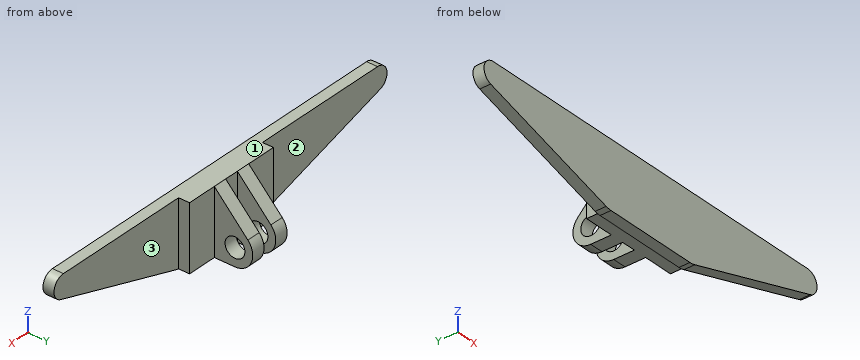
```python
from build123d import *

# Parameters (mm, degrees)
BOSS_EXTRUDE1_DEPTH = 6.9215
FILLET1_R           = 12.7
SKETCH2_W           = 63.5635
SKETCH2_H           = 41.073046068
BOSS_EXTRUDE2_DEPTH = 6.9215
SKETCH3_R           = 6.223
BOSS_EXTRUDE4_DEPTH = 44.7929
SKETCH3_2_R         = 6.223
CUT_EXTRUDE1_DEPTH  = 18.7706
SKETCH4_W           = 8.89
SKETCH4_H           = 24.13
CUT_EXTRUDE2_DEPTH  = 42.2115


with BuildPart() as part:
    # Sketch1 → Boss-Extrude1 (new body)
    with BuildSketch(Plane(origin=(0, 0, 0), x_dir=(1, 0, 0), z_dir=(0, 1, 0))):
        with BuildLine():
            Line((5.071738793, 14.002525941), (94.4245, 41.2115))
            Line((94.4245, 41.2115), (157.988, 41.2115))
            Line((157.988, 41.2115), (247.340761207, 14.002525941))
            ThreePointArc((247.340761207, 14.002525941), (252.334481209, 6.102605506), (245.25605, 0))
            Line((245.25605, 0), (7.15645, 0))
            ThreePointArc((7.15645, 0), (0.078018791, 6.102605506), (5.071738793, 14.002525941))
        make_face()
    extrude(amount=BOSS_EXTRUDE1_DEPTH)

    # Fillet1
    fillet1_edges = [part.edges().sort_by_distance(p)[0] for p in [
        (94.4245, 3.46075, -41.2115),
        (157.988, 3.46075, -41.2115),
    ]]
    fillet(fillet1_edges, radius=FILLET1_R)

    # Sketch2 → Boss-Extrude2 (add)
    with BuildSketch(Plane(origin=(0, 6.9215, 0), x_dir=(1, 0, 0), z_dir=(0, 1, 0))):
        with Locations((126.226863171, 20.536523034)):
            Rectangle(SKETCH2_W, SKETCH2_H)
    extrude(amount=BOSS_EXTRUDE2_DEPTH)

    # Sketch3 → Boss-Extrude4 (add)
    with BuildSketch(Plane.ZY.offset(-94.445113171)):
        with BuildLine():
            Line((-41.073046068, 26.8097), (-41.073046068, 13.843))
            Line((-41.073046068, 13.843), (0, 13.843))
            Line((0, 13.843), (-22.230594652, 34.912162614))
            ThreePointArc((-22.230594652, 34.912162614), (-34.319655131, 37.065038558), (-41.073046068, 26.8097))
        make_face()
        with Locations((-29.909746068, 26.8097)):
            Circle(SKETCH3_R, mode=Mode.SUBTRACT)
    extrude(amount=-BOSS_EXTRUDE4_DEPTH)

    # Sketch3<2> → Cut-Extrude1 (cut)
    with BuildSketch(Plane.ZY.offset(-94.445113171)):
        with BuildLine():
            Line((-41.073046068, 26.8097), (-41.073046068, 13.843))
            Line((-41.073046068, 13.843), (0, 13.843))
            Line((0, 13.843), (-22.230594652, 34.912162614))
            ThreePointArc((-22.230594652, 34.912162614), (-34.319655131, 37.065038558), (-41.073046068, 26.8097))
        make_face()
        with Locations((-29.909746068, 26.8097)):
            Circle(SKETCH3_2_R, mode=Mode.SUBTRACT)
    extrude(amount=-CUT_EXTRUDE1_DEPTH, mode=Mode.SUBTRACT)

    # Sketch4 → Cut-Extrude2 (cut, through all)
    with BuildSketch(Plane.XY):
        with Locations((126.226863171, 25.908)):
            Rectangle(SKETCH4_W, SKETCH4_H)
    extrude(amount=-CUT_EXTRUDE2_DEPTH, mode=Mode.SUBTRACT)


solid = part.part
```
Geometry: final body of the model. Coordinates: model frame, mm. Face numbers are marked on the shaded views. A direction names the side the tool comes from. Round coordinates to 2 decimals unless told otherwise and drop trailing zeros. Write each loop counter-clockwise with the first axis right and the second up, starting at its lowest first coordinate (ties: lowest second). Pieces come first, ordered by that corner, then holes. Notation, with made-up numbers: (44, 79) -> (95, 79) arc R27 cw to (95, 105) -> close; hole circle Ø11 at (46, 82). An arc over 180 degrees is marked (long way). Return JSON: item names as keys, results as strings.
Q1. Section A-A on x = 119. Return the cut outline in (y, z), and give its area (3 significant figures).
From the geometry:
{"outline": "(0, -41.21) -> (6.92, -41.21) -> (6.92, -41.07) -> (26.81, -41.07) arc R11.16 ccw to (34.91, -22.23) -> (13.84, 0) -> (0, 0) -> close; hole circle Ø12.45 at (26.81, -29.91)", "area": "1,100 mm2"}
Q2. First-contact query: pin 1 Ø12 at (y, z) = (15, -31.5) entering from -X; pin 2 Ø16 at (y, z) = (26.81, -29.91) entering from -X; pin 3 Ø5 at (x, z) = (138, -8.5) entering from +Y. Flat tips, straight axial feed; report the tip coordinate or a pass-through.
From the geometry:
{"pin 1": "x = 94.45", "pin 2": "x = 113.22", "pin 3": "y = 24.27"}
Q3. Section D-D on y = 29. Return the cut outline in (x, z).
From the geometry:
{"outline": "(113.22, -40.86) -> (121.78, -40.86) -> (121.78, -35.73) -> (113.22, -35.73) -> close; (113.22, -24.08) -> (121.78, -24.08) -> (121.78, -15.99) -> (113.22, -15.99) -> close; (130.67, -40.86) -> (139.24, -40.86) -> (139.24, -35.73) -> (130.67, -35.73) -> close; (130.67, -24.08) -> (139.24, -24.08) -> (139.24, -15.99) -> (130.67, -15.99) -> close"}
Q4. Set-up query: the marked faces 1, 2 and 3. Return all of +Z, -Z, +X, -X, +Y, -Y with unobstructed straight access to the full face (end or side cutting, diameter ignored); none if empty.
From the geometry:
{"face 1": "+Z, +X, -X, +Y, -Y", "face 2": "+Z, -Z, -X, +Y", "face 3": "+Z, -Z, +X, +Y"}
Q5. Ray query, line 1 (X direction, y = 18.5, z = -29); line 2 (Y direction, x = 150, z = -4); line 3 (Y direction, x = 184, z = -26). Return the intervals inside material, ascending.
From the geometry:
{"line 1": "113.22 to 121.78, 130.67 to 139.24", "line 2": "0 to 13.84", "line 3": "0 to 6.92"}
Q6. Section C-C on z = -30. Return the cut outline in (x, y), and give its area (3 significant figures).
From the geometry:
{"outline": "(57.61, 0) -> (194.81, 0) -> (194.81, 6.92) -> (158.01, 6.92) -> (158.01, 13.84) -> (139.24, 13.84) -> (139.24, 20.59) -> (130.67, 20.59) -> (130.67, 13.84) -> (121.78, 13.84) -> (121.78, 20.59) -> (113.22, 20.59) -> (113.22, 13.84) -> (94.45, 13.84) -> (94.45, 6.92) -> (57.61, 6.92) -> close; (113.22, 33.03) -> (121.78, 33.03) -> (121.78, 37.97) -> (113.22, 37.97) -> close; (130.67, 33.03) -> (139.24, 33.03) -> (139.24, 37.97) -> (130.67, 37.97) -> close", "area": "1,590 mm2"}
Q7. Section B-B on y = 17.5. Return the cut outline in (x, z).
From the geometry:
{"outline": "(113.22, -41.07) -> (121.78, -41.07) -> (121.78, -3.86) -> (113.22, -3.86) -> close; (130.67, -41.07) -> (139.24, -41.07) -> (139.24, -3.86) -> (130.67, -3.86) -> close"}
